```python
from build123d import *

# Parameters (mm, degrees)
BOSS_EXTRUDE1_DEPTH = 6
BOSS_EXTRUDE2_DEPTH = 2.5
FILLET1_R           = 4
SKETCH3_R           = 2
CUT_EXTRUDE1_DEPTH  = 96.713112999
SKETCH4_R           = 2
CUT_EXTRUDE2_DEPTH  = 5


with BuildPart() as part:
    # Sketch1 → Boss-Extrude1 (new, symmetric)
    with BuildSketch(Plane.XY):
        Polygon((-49, 0), (-34.781308697, 0), (-20.781308697, 82), (20.781308697, 82), (34.781308697, 0), (49, 0), (49, 5), (39, 5), (25, 87), (-25, 87), (-39, 5), (-49, 5), align=None)
    extrude(amount=BOSS_EXTRUDE1_DEPTH, both=True)

    # Sketch2 → Boss-Extrude2 (add, symmetric)
    with BuildSketch(Plane.XY):
        with BuildLine():
            Line((31.450240635, 19.510541506), (27.939451789, 40.073733316))
            ThreePointArc((27.939451789, 40.073733316), (0.037609002, 49.999938394), (-27.914924838, 40.217391174))
            Line((-27.914924838, 40.217391174), (-31.357853442, 20.051666495))
            ThreePointArc((-31.357853442, 20.051666495), (0.220379798, 39.998805231), (31.450240635, 19.510541506))
        make_face()
    extrude(amount=BOSS_EXTRUDE2_DEPTH, both=True)

    # Fillet1
    fillet1_edges = [part.edges().sort_by_distance(p)[0] for p in [
        (27.939451789, 40.073733316, 0),
        (-27.914924838, 40.217391174, 0),
    ]]
    fillet(fillet1_edges, radius=FILLET1_R)

    # Sketch3 → Cut-Extrude1 (cut, through all)
    with BuildSketch(Plane(origin=(0, 5, 0), x_dir=(1, 0, 0), z_dir=(0, 1, 0))):
        with Locations(Location((-44, 0, 0), (0, 0, 180))):
            Circle(SKETCH3_R)
        with Locations(Location((44, 0, 0), (0, 0, 180))):
            Circle(SKETCH3_R)
    extrude(amount=-CUT_EXTRUDE1_DEPTH, mode=Mode.SUBTRACT)

    # Sketch4 → Cut-Extrude2 (cut)
    with BuildSketch(Plane(origin=(0, 87, 0), x_dir=(1, 0, 0), z_dir=(0, 1, 0))):
        with Locations(Location((-20, 0, 0), (0, 0, 270))):
            Circle(SKETCH4_R)
        with Locations(Location((20, 0, 0), (0, 0, 270))):
            Circle(SKETCH4_R)
    extrude(amount=-CUT_EXTRUDE2_DEPTH, mode=Mode.SUBTRACT)


solid = part.part
```
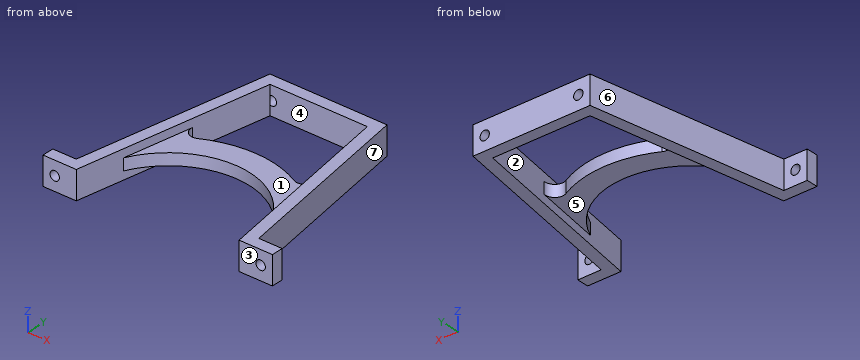
The listing builds one solid part. Answer for the finished solid, in the listing's coordinates (mm). Face numbers are marked on the shaded views. A direction names the side the tool comes from. Round coordinates to 2 decimals unless told otherwise and drop trailing zeros. Loops run counter-clockwise (first coordinate to the right, second up) from the corner with the lowest first, then second, coordinate; pieces in that order, holes last. Notation, with made-up numbers: (19.25, 2.5) - (62.25, 2.5) arc R16 cw to (62.25, 24.5) - close; hole circle Ø3 at (52.25, 38.5). An arc over 180 degrees is marked (long way). Return JSON: item names as keys, results as strings. Group by question number.
1. Each of these flat-tipped pins is pushed along its axis until it touches: P1, Ø3, axis at x = 42.5, z = 2, coming from the +Y side; P2, Ø3.5, axis at x = 20, z = 0, coming from the +Y side; P3, Ø1, axis at x = -20.5, y = 39, coming from the -Z side; P4, Ø3, axis at x = 44, z = 0, coming from the -Y side. Where does it stop, or does it pass through?
2. Consider probe 1 along Z at (x, y) = (-44, 2); probe 2 along X at (y, z) = (45.5, 0); probe 3 along X at (y, z) = (84.6, 0). Determine where each line is inside the solid, lowest interval first.
3. The mould has two halves that part along X. Classify the marked faces 5, 6 and 7: pulls with the +X half, pulls with the -X half, needs draft (parallel to the pull), parting line crosses it, or undercut.
4. The part is cut by section B-B on z = 0. State how many separate pieces and enclosed holes the cut face has, then the cut area to 3 significant figures.
5. Which of the six approach directions +Z, -Z, +X, -X, +Y, -Y give full straight-line access (tool end or side, diameter ignored) to the marked faces 1, 2, 3 and 4?
6. The part is cut by section C-C on y = 11. Determine the outline of the cut face in (x, z).
7. The part is cut by section A-A on x = 44. Determine the outline of the cut face in (y, z).
Resolved:
{
 "1": {"P1": "stops at y = 5", "P2": "stops at y = 82", "P3": "stops at z = -2.5", "P4": "passes through"},
 "2": {"probe 1": "z = -6 to -2, 2 to 6", "probe 2": "x = -32.09 to -25.04, -19.58 to 19.42, 25.15 to 32.09", "probe 3": "x = -25.41 to -22, -18 to 18, 22 to 25.41"},
 "3": {"face 5": "undercut", "face 6": "pulls with the -X half", "face 7": "pulls with the +X half"},
 "4": {"separate pieces": "4", "enclosed holes": "0", "area": "1,810 mm²"},
 "5": {"face 1": "+Z, -Y", "face 2": "none", "face 3": "+Z, -Z, +X, -X, -Y", "face 4": "+Z, -Z"},
 "6": {"outline": "(-37.98, -6) - (-32.9, -6) - (-32.9, 6) - (-37.98, 6) - close; (32.9, -6) - (37.98, -6) - (37.98, 6) - (32.9, 6) - close"},
 "7": {"outline": "(0, -6) - (5, -6) - (5, -2) - (0, -2) - close; (0, 2) - (5, 2) - (5, 6) - (0, 6) - close"}
}
